Can you work these out from the model? Positions are in its coordinate system, mm. Round coordinates to 2 decimals unless told otherwise and drop trailing zeros. Write each loop counter-clockwise with the first axis right and the second up, starting at its lowest first coordinate (ties: lowest second). Pieces come first, ordered by that corner, then holes. Notation, with made-up numbers: (12, 71.25) - (44, 71.25) arc R21 cw to (44, 83.25) - close; hole circle Ø7 at (-21.5, 12.25). An arc over 180 degrees is marked (long way). One line per item, written item: value. Start each with the question number.
(1) I want a section at A-A on z = -9. List the corners of the cut face in (x, y) for me.
(2) I want a section at C-C on y = 1.65. Give the number of separate pieces and of enclosed holes in the cut face, plus the area to 3 significant figures.
(3) I want a section at B-B on x = -3. List the corners of the cut face in (y, z) for me.
(4) Thinking about a two-plate mould opening in Z: for faces 1 (the face through (-11.27, 1.479, 3.683)), 2 (the face through (0, 0, -17)), which applies, +Z half, -Z half, draft (parallel to the pull), parting line (faces both ways), or undercut?
(5) I'm going to push a flat-ended pin straight in: pin 1 Ø1 at (x, y) = (-2, 2) entering from -Z. Where does the tip first touch, or does it pass through?
(6) I want a section at D-D on z = -25.3. List the corners of the cut face in (x, y) for me, plus the area to 3 significant figures.
(7) If I drill on L1, parallel to Z at x = 15.5, y = 0.8; L2, parallel to X at y = 0.65, z = -6.5; L3, parallel to Z at x = -2, y = 0.9, over which ranges is the centre line in solid material (lowest first)? Write a range as from..to.
from build123d import *

# Parameters (mm, degrees)
SKETCH_1_R               = 4.2
EXTRUDE_1_DEPTH          = 3
CUT_EXTRUDE_1_DEPTH      = 44.0464865
CUT_EXTRUDE_1_DEPTH_BACK = 44.0464865
SKETCH_2_W               = 16
SKETCH_2_H               = 20
FILLET_1_R               = 2


with BuildPart() as part:
    # Sketch 1 → Extrude 1 (new body)
    with BuildSketch(Plane(origin=(0, 0, 0), x_dir=(1, 0, 0), z_dir=(0, 1, 0))):
        with BuildLine():
            ThreePointArc((20, 18), (0, 38), (-20, 18))
            Line((-20, 18), (-20, -18))
            Line((-20, -18), (20, -18))
            Line((20, -18), (20, 18))
        make_face()
        with Locations(Location((0, 25.3, 0), (0, 0, 270))):
            Circle(SKETCH_1_R, mode=Mode.SUBTRACT)
        with BuildLine():
            Line((15.3, 6), (15.3, -2))
            ThreePointArc((15.3, -2), (16.007106781, -3.707106781), (14.3, -3))
            Line((14.3, -3), (13, -3))
            ThreePointArc((13, -3), (11.292893219, -3.707106781), (12, -2))
            Line((12, -2), (12, 6))
            ThreePointArc((12, 6), (11.292893219, 7.707106781), (13, 7))
            Line((13, 7), (14.3, 7))
            ThreePointArc((14.3, 7), (16.007106781, 7.707106781), (15.3, 6))
        make_face(mode=Mode.SUBTRACT)
        with BuildLine():
            Line((-12, 6), (-12, -2))
            ThreePointArc((-12, -2), (-11.292893219, -3.707106781), (-13, -3))
            Line((-13, -3), (-14.3, -3))
            ThreePointArc((-14.3, -3), (-16.007106781, -3.707106781), (-15.3, -2))
            Line((-15.3, -2), (-15.3, 6))
            ThreePointArc((-15.3, 6), (-16.007106781, 7.707106781), (-14.3, 7))
            Line((-14.3, 7), (-13, 7))
            ThreePointArc((-13, 7), (-11.292893219, 7.707106781), (-12, 6))
        make_face(mode=Mode.SUBTRACT)
        with BuildLine():
            Line((-7.65, -12), (-7.65, -10.7))
            ThreePointArc((-7.65, -10.7), (-8.357106781, -8.992893219), (-6.65, -9.7))
            Line((-6.65, -9.7), (6.65, -9.7))
            ThreePointArc((6.65, -9.7), (8.357106781, -8.992893219), (7.65, -10.7))
            Line((7.65, -10.7), (7.65, -12))
            ThreePointArc((7.65, -12), (8.357106781, -13.707106781), (6.65, -13))
            Line((6.65, -13), (-6.65, -13))
            ThreePointArc((-6.65, -13), (-8.357106781, -13.707106781), (-7.65, -12))
        make_face(mode=Mode.SUBTRACT)
    extrude(amount=EXTRUDE_1_DEPTH)

    # Sketch 2 → Cut-Extrude 1 (cut, two sides: drawn at the far end of the back side and taken through both)
    with BuildSketch(Plane(origin=(0, 3, 0), x_dir=(1, 0, 0), z_dir=(0, 1, 0)).offset(-CUT_EXTRUDE_1_DEPTH_BACK)):
        with Locations((0, 4)):
            Rectangle(SKETCH_2_W, SKETCH_2_H)
    extrude(amount=CUT_EXTRUDE_1_DEPTH + CUT_EXTRUDE_1_DEPTH_BACK, mode=Mode.SUBTRACT)

    # Fillet 1
    fillet_1_edges = [part.edges().sort_by_distance(p)[0] for p in [
        (8, 1.5, -14),
        (8, 1.5, 6),
        (-8, 1.5, 6),
        (-8, 1.5, -14),
    ]]
    fillet(fillet_1_edges, radius=FILLET_1_R)


solid = part.part
Established:
1. outline: (-20, 0) - (-8, 0) - (-8, 3) - (-20, 3) - close; (8, 0) - (20, 0) - (20, 3) - (8, 3) - close
2. separate pieces: 1
2. enclosed holes: 5
2. area: 1,550 mm2
3. outline: (0, -37.77) - (3, -37.77) - (3, -28.24) - (0, -28.24) - close; (0, -22.36) - (3, -22.36) - (3, -14) - (0, -14) - close; (0, 6) - (3, 6) - (3, 9.7) - (0, 9.7) - close; (0, 13) - (3, 13) - (3, 18) - (0, 18) - close
4. face 1: undercut
4. face 2: draft
5. pin 1: z = -37.94
6. outline: (-18.62, 0) - (-4.2, 0) - (-4.2, 3) - (-18.62, 3) - close; (4.2, 0) - (18.62, 0) - (18.62, 3) - (4.2, 3) - close
6. area: 86.5 mm2
7. L1: -30.64..-7.98, -6.02..2.02, 3.98..18
7. L2: -20..-16.17, -11.13..-8, 8..11.13, 16.17..20
7. L3: -37.9..-28.99, -21.61..-14, 6..9.7, 13..18
